Design review of the part built by this model. Coordinates are the model's own, in mm. A direction names the side the tool comes from. Give positions to 0.01 mm unless a question says otherwise; leave off trailing zeros. Loops run counter-clockwise (first coordinate to the right, second up) from the corner with the lowest first, then second, coordinate; pieces in that order, holes last. Notation, with made-up numbers: (-35.5, -14.5) -> (-7.5, -14.5) arc R29 cw to (-7.5, 6.5) -> close; hole circle Ø1 at (12.25, 85.25). An arc over 180 degrees is marked (long way). Answer as CSV lines item,"result".
from build123d import *

# Parameters (mm, degrees)
F0_W     = 70.3
F0_H     = 58.1155021116
F1_DEPTH = 4.7
F2_DEPTH = 2.7
F0_H_2   = 4
F0_H_3   = 4.7
F3_DEPTH = 2.7


# Not quite as in the source:
# - a feature names something its author has since deleted; it is built from what else it names


with BuildPart() as f1:
    # F0 (on Top) → F1 (new body)
    with BuildSketch(Plane.XY):
        Polygon((0, -2), (0, 0), (0, 2), (-4.7, 2), (-4.7, -2), (-4.7, -60.1155021116), (-4.7, -64.1155021116), (0, -64.1155021116), (0, -62.1155021116), (0, -60.1155021116), align=None)
        Polygon((0, 2), (0, 0), (0, -2), (0, -60.1155021116), (0, -62.1155021116), (0, -64.1155021116), (4.7, -64.1155021116), (4.7, -60.1155021116), (4.7, -2), (4.7, 2), align=None)
        Polygon((-4.7, 2), (0, 2), (0, 132.9871674252), (-4.9, 132.9871674252), (-75, 2), align=None)
        Polygon((0, 132.9871674252), (0, 2), (4.7, 2), (75, 2), (4.9, 132.9871674252), align=None)
        with Locations((-39.85, -31.0577510558)):
            Rectangle(F0_W, F0_H)
        with Locations((39.85, -31.0577510558)):
            Rectangle(F0_W, F0_H)
        Polygon((4.7, -64.1155021116), (0, -64.1155021116), (0, -124.2310042232), (4.7, -124.2310042232), (4.7, -119.5310042232), (75, -119.5310042232), (75, -64.1155021116), align=None)
        Polygon((0, -124.2310042232), (0, -64.1155021116), (-4.7, -64.1155021116), (-75, -64.1155021116), (-75, -119.5310042232), (-4.7, -119.5310042232), (-4.7, -121.7700988054), (-4.7, -124.2310042232), align=None)
    extrude(amount=F1_DEPTH)

    # F0 (on Top) → F2 (join)
    with BuildSketch(Plane.XY):
        Polygon((-4.7, -2), (-4.7, 2), (-75, 2), (-75, 0), (-75, -2), align=None)
        Polygon((75, 2), (4.7, 2), (4.7, -2), (75, -2), (75, 0), align=None)
    extrude(amount=F2_DEPTH)

    # F0 (on Top) → F3 (join)
    with BuildSketch(Plane.XY):
        with Locations((-39.85, -62.1155021116)):
            Rectangle(F0_W, F0_H_2)
        with Locations((39.85, -62.1155021116)):
            Rectangle(F0_W, F0_H_2)
        Polygon((75, 2), (4.7, 2), (4.7, -2), (75, -2), (75, 0), align=None)
        Polygon((-75, -124.2310042232), (-4.7, -124.2310042232), (-4.7, -121.7700988054), (-4.7, -119.5310042232), (-75, -119.5310042232), align=None)
        with Locations((39.85, -121.8810042232)):
            Rectangle(F0_W, F0_H_3)
    extrude(amount=F3_DEPTH)


solid = f1.part
Q1. We need section C-C, the plane y = 75. State the section outline as (x, z) points.
Filled sheet:
outline,"(-35.93, 0) -> (35.93, 0) -> (35.93, 4.7) -> (-35.93, 4.7) -> close"
Q2. For faces 1 (the flat face through (39, -122, 2.7)), 2 (the flat face through (-40, -122, 2.7)), 3 (the flat face through (-75, -62, 2)), list the 3-axis set-ups (+Z, -Z, +X, -X, +Y, -Y) from which the entire face can be reached by the end or side of a thin tool; tool diameter is ignored.
Filled sheet:
face 1,"+Z, +X, -Y"
face 2,"+Z, -X, -Y"
face 3,"+Z, -Z, -X, +Y, -Y"
Q3. To check wall thickness, follow probe 1 along Y at (x, z) = (-39, 4.25); probe 2 along Y at (x, z) = (13, 4.1); probe 3 along Y at (x, z) = (49.5, 1.1). State the ranges of each line that lie inside material, in increasing order. Write a range as from..to.
Filled sheet:
probe 1,"y = -119.53..-64.12, -60.12..-2, 2..69.27"
probe 2,"y = -119.53..-64.12, -60.12..-2, 2..117.85"
probe 3,"y = -124.23..49.65"
Q4. We need section B-B, the plane x = 28. State the section outline as (y, z) points.
Filled sheet:
outline,"(-124.23, 0) -> (89.82, 0) -> (89.82, 4.7) -> (2, 4.7) -> (2, 2.7) -> (-2, 2.7) -> (-2, 4.7) -> (-60.12, 4.7) -> (-60.12, 2.7) -> (-64.12, 2.7) -> (-64.12, 4.7) -> (-119.53, 4.7) -> (-119.53, 2.7) -> (-124.23, 2.7) -> close"
Q5. We need section A-A, the plane z = 3.7. State the section outline as (x, y) points.
Filled sheet:
outline,"(-75, -119.53) -> (-4.7, -119.53) -> (-4.7, -124.23) -> (4.7, -124.23) -> (4.7, -119.53) -> (75, -119.53) -> (75, -64.12) -> (4.7, -64.12) -> (4.7, -60.12) -> (75, -60.12) -> (75, -2) -> (4.7, -2) -> (4.7, 2) -> (75, 2) -> (4.9, 132.99) -> (-4.9, 132.99) -> (-75, 2) -> (-4.7, 2) -> (-4.7, -2) -> (-75, -2) -> (-75, -60.12) -> (-4.7, -60.12) -> (-4.7, -64.12) -> (-75, -64.12) -> close"
Q6. We need section D-D, the plane x = 66. State the section outline as (y, z) points, and give its area (3 significant figures).
Filled sheet:
outline,"(-124.23, 0) -> (18.82, 0) -> (18.82, 4.7) -> (2, 4.7) -> (2, 2.7) -> (-2, 2.7) -> (-2, 4.7) -> (-60.12, 4.7) -> (-60.12, 2.7) -> (-64.12, 2.7) -> (-64.12, 4.7) -> (-119.53, 4.7) -> (-119.53, 2.7) -> (-124.23, 2.7) -> close"
area,"647 mm^2"
Q7. Clearance check with flat-ended pins moving along their axes: pin 1 Ø1 at (y, z) = (-1, 3.5) entering from -X; pin 2 Ø1 at (y, z) = (-121, 3.5) entering from +X; pin 3 Ø1 at (x, z) = (-52, 3.5) entering from +Y. State where each tip first meets the part, or that it passes through.
Filled sheet:
pin 1,"stops at x = -4.7"
pin 2,"stops at x = 4.7"
pin 3,"stops at y = 45.91"
